Could you check a few things on this model? Use its own coordinates, in mm. Face numbers are marked on the shaded views. A direction names the side the tool comes from. Coordinates: 2 decimals unless noted, no trailing zeros. Write each loop counter-clockwise with the first axis right and the second up, starting at its lowest first coordinate (ties: lowest second). Pieces come first, ordered by that corner, then holes.
```python
from build123d import *

# Parameters (mm, degrees)
SKETCH1_W           = 19
SKETCH1_H           = 10
BOSS_EXTRUDE1_DEPTH = 10
SKETCH2_W           = 17
SKETCH2_H           = 8
CUT_EXTRUDE1_DEPTH  = 12
SKETCH3_W           = 13
SKETCH3_H           = 10.51996768
CUT_EXTRUDE3_DEPTH  = 8


with BuildPart() as part:
    # Sketch1 → Boss-Extrude1 (new body)
    with BuildSketch(Plane.XY):
        with Locations((-0.130136986, 2.22260274)):
            Rectangle(SKETCH1_W, SKETCH1_H)
    extrude(amount=BOSS_EXTRUDE1_DEPTH)

    # Sketch2 → Cut-Extrude1 (cut)
    with BuildSketch(Plane.XY.offset(10)):
        with Locations((-0.130136986, 2.22260274)):
            Rectangle(SKETCH2_W, SKETCH2_H)
    extrude(amount=-CUT_EXTRUDE1_DEPTH, mode=Mode.SUBTRACT)

    # Sketch3 → Cut-Extrude3 (cut)
    with BuildSketch(Plane.XY):
        with Locations((-0.130136986, 2.34516547)):
            Rectangle(SKETCH3_W, SKETCH3_H)
    extrude(amount=CUT_EXTRUDE3_DEPTH, mode=Mode.SUBTRACT)


solid = part.part
```
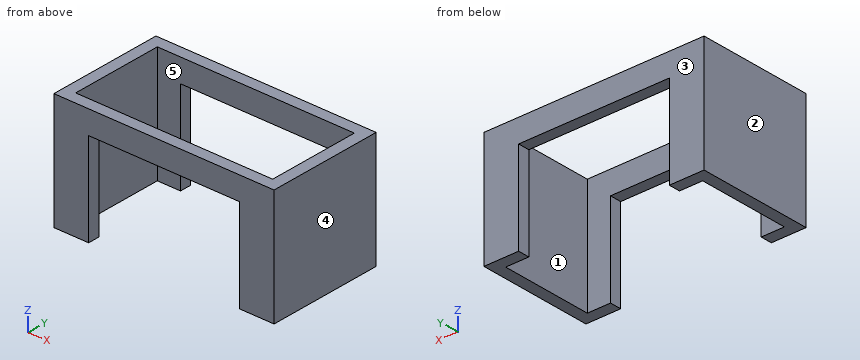
1. If we mould it in two halves opening along Y, with no side actions, what happens to the marked faces 3, 4 and 5? For each: pulls with the +Y half, pulls with the -Y half, needs draft (parallel to the pull), parting line crosses it, or undercut.
Verdict:
face 3: pulls with the +Y half
face 4: needs draft
face 5: undercut
2. I want a section at D-D on y = -2. Please give me the cut outline in (x, z).
Verdict:
outline: (-9.63, 0) - (-6.63, 0) - (-6.63, 8) - (6.37, 8) - (6.37, 0) - (9.37, 0) - (9.37, 10) - (-9.63, 10) - close
3. For pin 1 (0.8 mm diameter, centred on x = -1.5, y = -2.5, fed in from -Z), with a flat end and sliding along its axis, tell me the tip position at first contact or that it passes through.
Verdict:
pin 1: stops at z = 8
4. I want a section at A-A on x = -4.25. Please give me the cut outline in (y, z).
Verdict:
outline: (-2.78, 8) - (-1.78, 8) - (-1.78, 10) - (-2.78, 10) - close; (6.22, 8) - (7.22, 8) - (7.22, 10) - (6.22, 10) - close
5. Please list where these lines run through material, in increasing order: line 1 along X through (y, z) = (3, 3.25); line 2 along Y through (x, z) = (7, 2.25); line 3 along X through (y, z) = (6.75, 7.75).
Verdict:
line 1: x = -9.63 to -8.63, 8.37 to 9.37
line 2: y = -2.78 to -1.78, 6.22 to 7.22
line 3: x = -9.63 to -6.63, 6.37 to 9.37
6. On a 3-axis mill with a long thin cutter (end or side, diameter ignored), from which of +Z, -Z, +X, -X, +Y, -Y can I reach the whole of each face in a straight line? I mean the marked faces 1 and 2. Say none if no direction works.
Verdict:
face 1: +Z, -Z
face 2: +Z, -Z, -X, +Y, -Y
7. I want a section at C-C on y = 6. Please give me the cut outline in (x, z), plus the area to 3 significant figures.
Verdict:
outline: (-9.63, 0) - (-8.63, 0) - (-8.63, 10) - (-9.63, 10) - close; (8.37, 0) - (9.37, 0) - (9.37, 10) - (8.37, 10) - close
area: 20.0 mm2
8. I want a section at B-B on z = 6.5. Please give me the cut outline in (x, y).
Verdict:
outline: (-9.63, -2.78) - (-6.63, -2.78) - (-6.63, -1.78) - (-8.63, -1.78) - (-8.63, 6.22) - (-6.63, 6.22) - (-6.63, 7.22) - (-9.63, 7.22) - close; (6.37, -2.78) - (9.37, -2.78) - (9.37, 7.22) - (6.37, 7.22) - (6.37, 6.22) - (8.37, 6.22) - (8.37, -1.78) - (6.37, -1.78) - close
